from build123d import *

# Parameters (mm, degrees)
F1_DEPTH = 38.1


with BuildPart() as f1:
    # F0 (on Top) → F1 (new body)
    with BuildSketch(Plane.XY):
        with BuildLine():
            Line((0, 88.9), (0, 0))
            Line((0, 0), (88.9, 0))
            Line((88.9, 0), (88.9, 29.757951))
            ThreePointArc((88.9, 29.757951), (85.03308, 49.198269), (74.021024, 65.678976))
            Line((74.021024, 65.678976), (65.678976, 74.021024))
            ThreePointArc((65.678976, 74.021024), (49.198269, 85.03308), (29.757951, 88.9))
            Line((29.757951, 88.9), (0, 88.9))
        make_face()
        with BuildLine():
            Line((88.9, 0), (0, 0))
            Line((0, 0), (0, -88.9))
            Line((0, -88.9), (29.757951, -88.9))
            ThreePointArc((29.757951, -88.9), (49.198269, -85.03308), (65.678976, -74.021024))
            Line((65.678976, -74.021024), (74.021024, -65.678976))
            ThreePointArc((74.021024, -65.678976), (85.03308, -49.198269), (88.9, -29.757951))
            Line((88.9, -29.757951), (88.9, 0))
        make_face()
    extrude(amount=F1_DEPTH)


solid = f1.part
The model under review builds one solid part; all positions refer to its coordinate system, in mm. Give positions to 0.01 mm unless a question says otherwise; leave off trailing zeros. Loops run counter-clockwise (first coordinate to the right, second up) from the corner with the lowest first, then second, coordinate; pieces in that order, holes last. Notation, with made-up numbers: (78, 20.5) -> (120, 20.5) arc R14 ccw to (120, 27.5) -> close; hole circle Ø11 at (30, 48). An arc over 180 degrees is marked (long way). Put each result on its own line as item: value. Start each with the question number.
1. Wall thickness on probe 1 along X at (y, z) = (40.5, 21.5); probe 2 along X at (y, z) = (67, 26); probe 3 along Y at (x, z) = (33, 33): over which ranges is each line inside the solid? List them lowest first.
2. We need section B-B on x = 70.5. State the section outline as (y, z) points, then the cut area to 3 significant figures.
3. Clearance check with flat-ended pins moving along their axes: P1, Ø6, axis at y = -71, z = 6, coming from the +X side; P2, Ø12, axis at x = 52.5, z = 28.5, coming from the -Y side; P3, Ø8, axis at y = 59, z = 26.5, coming from the +X side. State where each tip first meets the part, or that it passes through.
4. We need section A-A on z = 4. State the section outline as (x, y) points, then the cut area to 3 significant figures.
5. Mouldability with a two-part tool opening along X and no side actions: class faces 1 (the face through (44, 1, 38.1)), 2 (the face through (85.14, 48.94, 18.78)), 3 (the face through (0, 1, 19)) as released by +X, released by -X, zero draft, split by the parting line, or undercut.
6. We need section C-C on y = -70. State the section outline as (x, z) points.
Determined:
1. probe 1: 0 to 87.75
1. probe 2: 0 to 72.7
1. probe 3: -88.8 to 88.8
2. outline: (-69.2, 0) -> (69.2, 0) -> (69.2, 38.1) -> (-69.2, 38.1) -> close
2. area: 5,270 mm^2
3. P1: x = 71.7
3. P2: y = -86.06
3. P3: x = 82.18
4. outline: (0, -88.9) -> (29.76, -88.9) arc R50.8 ccw to (65.68, -74.02) -> (74.02, -65.68) arc R50.8 ccw to (88.9, -29.76) -> (88.9, 29.76) arc R50.8 ccw to (74.02, 65.68) -> (65.68, 74.02) arc R50.8 ccw to (29.76, 88.9) -> (0, 88.9) -> close
4. area: 14,100 mm^2
5. face 1: zero draft
5. face 2: released by +X
5. face 3: released by -X
6. outline: (0, 0) -> (69.7, 0) -> (69.7, 38.1) -> (0, 38.1) -> close
